from build123d import *

# Parameters (mm, degrees)
SKETCH1_W           = 85
SKETCH1_H           = 90
BOSS_EXTRUDE1_DEPTH = 5
SKETCH2_W           = 60
SKETCH2_H           = 26.3
CUT_EXTRUDE2_DEPTH  = 7.5
SKETCH4_W           = 5
SKETCH4_H           = 26.3
CUT_EXTRUDE3_DEPTH  = 7.5
SKETCH5_W           = 30.2
SKETCH5_H           = 5
CUT_EXTRUDE4_DEPTH  = 5


with BuildPart() as part:
    # Sketch1 → Boss-Extrude1 (new body)
    with BuildSketch(Plane(origin=(0, 0, 0), x_dir=(1, 0, 0), z_dir=(0, 1, 0))):
        Rectangle(SKETCH1_W, SKETCH1_H)
    extrude(amount=BOSS_EXTRUDE1_DEPTH)

    # Sketch2 → Cut-Extrude2 (cut)
    with BuildSketch(Plane(origin=(0, 5, 0), x_dir=(1, 0, 0), z_dir=(0, 1, 0))):
        with Locations((0, -8.85)):
            Rectangle(SKETCH2_W, SKETCH2_H)
        Polygon((37.5, 24.3), (37, 24.3), (37, 35.4), (-37, 35.4), (-37, 24.3), (-37.5, 24.3), (-37.5, 18.3), (37.5, 18.3), align=None)
    extrude(amount=-CUT_EXTRUDE2_DEPTH, mode=Mode.SUBTRACT)

    # Sketch4 → Cut-Extrude3 (cut)
    with BuildSketch(Plane(origin=(0, 5, 0), x_dir=(1, 0, 0), z_dir=(0, 1, 0))):
        with Locations((-40, -8.85)):
            Rectangle(SKETCH4_W, SKETCH4_H)
        with Locations((40, -8.85)):
            Rectangle(SKETCH4_W, SKETCH4_H)
    extrude(amount=-CUT_EXTRUDE3_DEPTH, mode=Mode.SUBTRACT)

    # Sketch5 → Cut-Extrude4 (cut)
    with BuildSketch(Plane(origin=(0, 5, 0), x_dir=(1, 0, 0), z_dir=(0, 1, 0))):
        with Locations((0, -42.5)):
            Rectangle(SKETCH5_W, SKETCH5_H)
    extrude(amount=-CUT_EXTRUDE4_DEPTH, mode=Mode.SUBTRACT)


solid = part.part
Geometry: final body of the model. Coordinates: model frame, mm. A direction names the side the tool comes from. Give positions to 0.01 mm unless a question says otherwise; leave off trailing zeros. Write each loop counter-clockwise with the first axis right and the second up, starting at its lowest first coordinate (ties: lowest second). Pieces come first, ordered by that corner, then holes. Notation, with made-up numbers: (-29, -24) -> (3, -24) arc R17 cw to (3, -1) -> close; hole circle Ø8 at (15.5, 47). An arc over 180 degrees is marked (long way). Answer as a JSON object with one key per item and string values.
1. Cut plane A-A on x = -7. Output: boundary loops of the cut face in (y, z).
Ans:
{"outline": "(0, -45) -> (5, -45) -> (5, -35.4) -> (0, -35.4) -> close; (0, -18.3) -> (5, -18.3) -> (5, -4.3) -> (0, -4.3) -> close; (0, 22) -> (5, 22) -> (5, 40) -> (0, 40) -> close"}
2. Cut plane B-B on z = -27. Output: boundary loops of the cut face in (x, y), and give its area (3 significant figures).
Ans:
{"outline": "(-42.5, 0) -> (-37, 0) -> (-37, 5) -> (-42.5, 5) -> close; (37, 0) -> (42.5, 0) -> (42.5, 5) -> (37, 5) -> close", "area": "55.0 mm^2"}
3. Contact query for flat-ended pins moving along their axis: pin 1 (2.5 mm diameter, centred on y = 3.5, z = 4.5, fed in from +X); pin 2 (10 mm diameter, centred on x = -24.5, z = -10, fed in from -Y); pin 3 (1.5 mm diameter, centred on x = -5, y = 0.5, fed in from +Z); pin 4 (1.5 mm diameter, centred on y = 2, z = 11, fed in from -X). Output: stop coordinate, or through.
Ans:
{"pin 1": "stops at x = 37.5", "pin 2": "stops at y = 0", "pin 3": "stops at z = 40", "pin 4": "stops at x = -37.5"}
4. Cut plane D-D on y = 3.25. Output: boundary loops of the cut face in (x, z).
Ans:
{"outline": "(-42.5, -45) -> (42.5, -45) -> (42.5, -4.3) -> (37.5, -4.3) -> (37.5, 22) -> (42.5, 22) -> (42.5, 45) -> (15.1, 45) -> (15.1, 40) -> (-15.1, 40) -> (-15.1, 45) -> (-42.5, 45) -> (-42.5, 22) -> (-37.5, 22) -> (-37.5, -4.3) -> (-42.5, -4.3) -> close; hole (-37.5, -24.3) -> (-37, -24.3) -> (-37, -35.4) -> (37, -35.4) -> (37, -24.3) -> (37.5, -24.3) -> (37.5, -18.3) -> (-37.5, -18.3) -> close; hole (-30, -4.3) -> (30, -4.3) -> (30, 22) -> (-30, 22) -> close"}
5. Mould query, pull axis Z, two halves, no side actions, for faces 1 (the flat face through (-30, 3, 9)), 2 (the flat face through (0, 3, 40)), 3 (the flat face through (-1, 5, -11)). Classes: pulls with the +Z half, pulls with the -Z half, needs draft (parallel to the pull), parting line crosses it, or undercut.
Ans:
{"face 1": "undercut", "face 2": "pulls with the +Z half", "face 3": "needs draft"}
6. Access query for faces 4 (the flat face through (15.1, 3, 43)), 5 (the flat face through (-37.5, 3, 9)), 6 (the flat face through (37.5, 3, 9)), 7 (the flat face through (0, 3, -4.3)). Directions: +Z, -Z, +X, -X, +Y, -Y. A direction counts if a zero-diameter tool reaches every point of the face in a straight line with its end or side. Return the directions, or none.
Ans:
{"face 4": "+Z, +Y, -Y", "face 5": "-X, +Y, -Y", "face 6": "+X, +Y, -Y", "face 7": "+Y, -Y"}
7. Ray query, probe 1 along Z at (x, y) = (26, 2.05); probe 2 along Z at (x, y) = (9, 3.3); probe 3 along X at (y, z) = (2.7, -32.5). Return the intervals inside material, ascending. Write a range as from..to.
Ans:
{"probe 1": "z = -45..-35.4, -18.3..-4.3, 22..45", "probe 2": "z = -45..-35.4, -18.3..-4.3, 22..40", "probe 3": "x = -42.5..-37, 37..42.5"}
8. Cut plane C-C on x = 35. Output: boundary loops of the cut face in (y, z).
Ans:
{"outline": "(0, -45) -> (5, -45) -> (5, -35.4) -> (0, -35.4) -> close; (0, -18.3) -> (5, -18.3) -> (5, 45) -> (0, 45) -> close"}
